from build123d import *

# Parameters (mm, degrees)
F0_R     = 12.6166
F0_R_2   = 12.680328
F0_R_3   = 12.670482
F0_R_4   = 13.894295
F0_R_5   = 12.421427
F0_R_6   = 12.153085
F0_R_7   = 12.859931
F0_R_8   = 13.359293
F0_R_9   = 13.464332
F0_R_10  = 11.644387
F0_R_11  = 14.14438
F0_R_12  = 13.545297
F1_DEPTH = 12.7
F2_R     = 25.4
F3_SIZE  = 6.35


with BuildPart() as f1:
    # F0 (on Front) → F1 (new body)
    with BuildSketch(Plane.XZ):
        Polygon((-228.6, -152.085962), (228.6, -152.085962), (228.6, 101.914038), (76.2, 355.914038), (-76.2, 355.914038), (-228.6, 101.914038), align=None)
        with Locations((-182.22025, -80.14226)):
            Circle(F0_R, mode=Mode.SUBTRACT)
        with Locations((-77.011786, -80.14226)):
            Circle(F0_R_2, mode=Mode.SUBTRACT)
        with Locations((-182.22025, 53.524222)):
            Circle(F0_R_3, mode=Mode.SUBTRACT)
        with Locations((-77.011786, 53.524222)):
            Circle(F0_R_4, mode=Mode.SUBTRACT)
        with Locations((76.489076, -80.14226)):
            Circle(F0_R_5, mode=Mode.SUBTRACT)
        with Locations((169.624433, -80.14226)):
            Circle(F0_R_6, mode=Mode.SUBTRACT)
        with Locations((76.489076, 53.524222)):
            Circle(F0_R_7, mode=Mode.SUBTRACT)
        with Locations((169.624433, 53.524222)):
            Circle(F0_R_8, mode=Mode.SUBTRACT)
        with Locations((-36.480658, 152.696133)):
            Circle(F0_R_9, mode=Mode.SUBTRACT)
        with Locations((-36.480658, 319.994807)):
            Circle(F0_R_10, mode=Mode.SUBTRACT)
        with Locations((40.269773, 152.696133)):
            Circle(F0_R_11, mode=Mode.SUBTRACT)
        with Locations((40.269773, 319.994807)):
            Circle(F0_R_12, mode=Mode.SUBTRACT)
    extrude(amount=F1_DEPTH)

    # F2
    f2_edges = [f1.edges().sort_by_distance(p)[0] for p in [
        (76.2, -6.35, 355.914038),
        (-76.2, -6.35, 355.914038),
        (228.6, -6.35, 101.914038),
        (228.6, -6.35, -152.085962),
        (-228.6, -6.35, -152.085962),
        (-228.6, -6.35, 101.914038),
    ]]
    fillet(f2_edges, radius=F2_R)

    # F3
    f3_edges = [f1.edges().sort_by_distance(p)[0] for p in [
        (26.724477, -12.7, 319.994807),
        (-48.125045, -12.7, 319.994807),
        (-49.94499, -12.7, 152.696133),
        (26.125393, -12.7, 152.696133),
        (-90.906081, -12.7, 53.524222),
        (-194.890732, -12.7, 53.524222),
        (63.629145, -12.7, 53.524222),
        (156.26514, -12.7, 53.524222),
        (157.471348, -12.7, -80.14226),
        (64.067649, -12.7, -80.14226),
        (-89.692114, -12.7, -80.14226),
        (-194.83685, -12.7, -80.14226),
    ]]
    chamfer(f3_edges, length=F3_SIZE)


solid = f1.part
For this review, take the finished solid that the model builds, in its own axes (mm). Round coordinates to 2 decimals unless told otherwise and drop trailing zeros. Order: outer loops, then holes, each group sorted by start corner. A loop starts at its lowest first (then second) coordinate and runs counter-clockwise, first axis right, second up. Notation, with made-up numbers: (-7.5, -31) -> (51.5, -31) arc R21 ccw to (51.5, -20) -> close; hole circle Ø2 at (5, 63.5). An arc over 180 degrees is marked (long way). Write item = value, one per line. Start each with the question number.
1) The part is to be moulded in two halves that separate along Z. For faces 1 (the face through (155.279, -6.261, 224.115)), 2 (the face through (-3, -12.7, 49)), 3 (the face through (-71, -6.7, -91.7)), 4 (the face through (-3, -6, -152.086)), say which applies: +Z half, -Z half, draft (parallel to the pull), parting line (faces both ways), or undercut.
2) Take a section at A-A on y = -3. Count the separate pieces of the cut face and the enclosed holes in it, plus the area to 3 significant figures.
3) To check wall thickness, follow line 1 (Z direction, x = -46.5, y = -11.25); line 2 (X direction, y = -8.75, z = 41.5); line 3 (X direction, y = -10.25, z = 328). State the ranges of each line that lie inside material, in increasing order. Write a range as from..to.
4) Take a section at C-C on z = 279. State the section outline as (x, y) points.
Verdict:
q1.face_1 = +Z half
q1.face_2 = draft
q1.face_3 = undercut
q1.face_4 = -Z half
q2.separate_pieces = 1
q2.enclosed_holes = 12
q2.area = 187,000 mm2
q3.line_1 = -152.09..137.31, 168.09..306.83, 333.16..355.91
q3.line_2 = -228.6..-191.31, -173.14..-88.01, -66.02..67.09, 85.89..159.44, 179.81..228.6
q3.line_3 = -92.95..-49.81, -23.16..24.77, 55.77..92.95
q4.outline = (-122.35, -12.7) -> (122.35, -12.7) -> (122.35, 0) -> (-122.35, 0) -> close
